For this review, use the dimensioned drawing (mm, ordinates from the lowest corner) and the shaded views. Coordinates: 2 decimals unless noted, no trailing zeros. One line per item, written item: value.
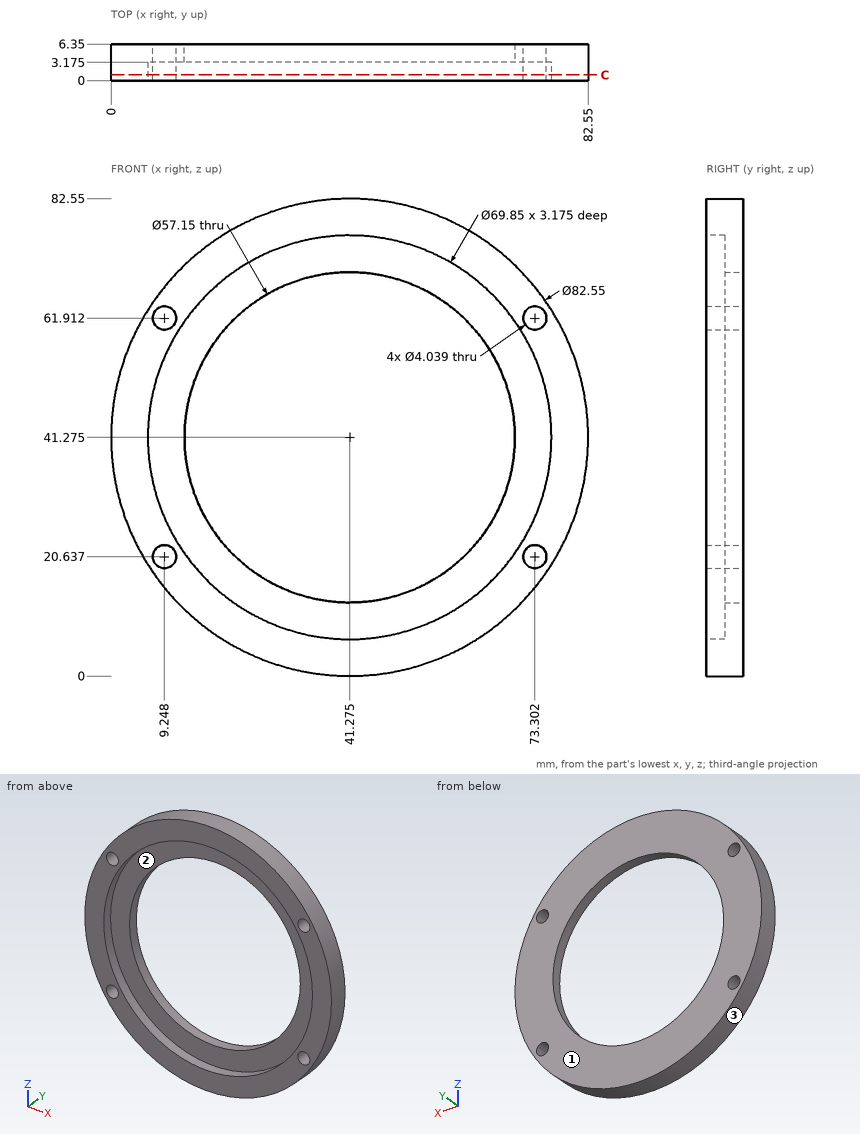
(1) Insertion check: pin 1 Ø1.5 at (x, z) = (15, 24.5) entering from -Y (1 decimal); pin 2 Ø3 at (x, y) = (44, 3.5) entering from +Z; pin 3 Ø1.5 at (x, y) = (54.5, 3.5) entering from -Z. Each pin has a flat end and moves straight along its axis. Give the tip position at first contact, or say it passes through.
Checks:
pin 1: y = 3.2
pin 2: z = 82.53
pin 3: z = 1.93
(2) To check wall thickness, follow L1, parallel to X at y = 4, z = 42; L2, parallel to Z at x = 34, y = 4 (1 decimal); L3, parallel to X at y = 1.5, z = 64 (1 decimal). State the ranges of each line that lie inside material, in increasing order. Write a range as [from, to].
Checks:
L1: [0.01, 12.71], [69.84, 82.54]
L2: [0.6, 13.6], [68.9, 81.9]
L3: [6.8, 14.8], [67.8, 75.7]
(3) Draft analysis for pull direction X (two halves, no side actions). For the marked faces 1, 2 and 3, state which applies: pulls with the +X half, pulls with the -X half, needs draft (parallel to the pull), parting line crosses it, or undercut.
Checks:
face 1: needs draft
face 2: undercut
face 3: parting line crosses it
(4) Add section C-C on y = 1. State how many separate pieces and enclosed holes the cut face has, then the cut area to 3 significant figures.
Checks:
separate pieces: 1
enclosed holes: 5
area: 1,470 mm^2
